```python
from build123d import *

# Parameters (mm, degrees)
SKETCH1_W             = 40
SKETCH1_H             = 30
BOSS_EXTRUDE1_DEPTH   = 400
BOSS_EXTRUDE1_2_DEPTH = 400
BOSS_EXTRUDE2_REACH   = 553.928
SKETCH2_W             = 40
SKETCH2_H             = 30
SKETCH3_W             = 40
SKETCH3_H             = 40
BOSS_EXTRUDE3_DEPTH   = 250
SKETCH4_W             = 40
SKETCH4_H             = 30
BOSS_EXTRUDE4_DEPTH   = 270
SKETCH5_W             = 40
SKETCH5_H             = 40
BOSS_EXTRUDE5_DEPTH   = 250
SKETCH6_W             = 40
SKETCH6_H             = 40
BOSS_EXTRUDE6_DEPTH   = 310


with BuildPart() as part:
    # Sketch1 → Boss-Extrude1 (new body)
    with BuildSketch(Plane.XY):
        Rectangle(SKETCH1_W, SKETCH1_H)
    extrude(amount=BOSS_EXTRUDE1_DEPTH)


with BuildPart() as body_2:
    # Sketch1 → Boss-Extrude1 2 (new body)
    with BuildSketch(Plane.XY):
        with Locations((380, 0)):
            Rectangle(SKETCH1_W, SKETCH1_H)
    extrude(amount=BOSS_EXTRUDE1_2_DEPTH)

    # Sketch2 → Boss-Extrude2 (add, up to next)
    with BuildSketch(Plane(origin=(20, 0, 0), x_dir=(0, 0, -1), z_dir=(1, 0, 0)), mode=Mode.PRIVATE) as boss_extrude2_sk1:
        with Locations((-380, 0)):
            Rectangle(SKETCH2_W, SKETCH2_H)
    boss_extrude2_tool1 = extrude(boss_extrude2_sk1.sketch, amount=BOSS_EXTRUDE2_REACH, mode=Mode.PRIVATE) - body_2.part
    # Sketch2 → Boss-Extrude2 (add, up to next)
    with BuildSketch(Plane(origin=(20, 0, 0), x_dir=(0, 0, -1), z_dir=(1, 0, 0)), mode=Mode.PRIVATE) as boss_extrude2_sk2:
        with Locations((-290, 0)):
            Rectangle(SKETCH2_W, SKETCH2_H)
    boss_extrude2_tool2 = extrude(boss_extrude2_sk2.sketch, amount=BOSS_EXTRUDE2_REACH, mode=Mode.PRIVATE) - body_2.part
    # Sketch2 → Boss-Extrude2 (add, up to next)
    with BuildSketch(Plane(origin=(20, 0, 0), x_dir=(0, 0, -1), z_dir=(1, 0, 0)), mode=Mode.PRIVATE) as boss_extrude2_sk3:
        with Locations((-110, 0)):
            Rectangle(SKETCH2_W, SKETCH2_H)
    boss_extrude2_tool3 = extrude(boss_extrude2_sk3.sketch, amount=BOSS_EXTRUDE2_REACH, mode=Mode.PRIVATE) - body_2.part
    # Sketch2 → Boss-Extrude2 (add, up to next)
    with BuildSketch(Plane(origin=(20, 0, 0), x_dir=(0, 0, -1), z_dir=(1, 0, 0)), mode=Mode.PRIVATE) as boss_extrude2_sk4:
        with Locations((-20, 0)):
            Rectangle(SKETCH2_W, SKETCH2_H)
    boss_extrude2_tool4 = extrude(boss_extrude2_sk4.sketch, amount=BOSS_EXTRUDE2_REACH, mode=Mode.PRIVATE) - body_2.part
    # Sketch2 → Boss-Extrude2 (add, up to next)
    with BuildSketch(Plane(origin=(20, 0, 0), x_dir=(0, 0, -1), z_dir=(1, 0, 0)), mode=Mode.PRIVATE) as boss_extrude2_sk5:
        with Locations((-200, 0)):
            Rectangle(SKETCH2_W, SKETCH2_H)
    boss_extrude2_tool5 = extrude(boss_extrude2_sk5.sketch, amount=BOSS_EXTRUDE2_REACH, mode=Mode.PRIVATE) - body_2.part

    add(part.part)  # Boss-Extrude2 merges part
    add(boss_extrude2_tool1.solids().sort_by_distance((20, 0, 380))[0])
    add(boss_extrude2_tool2.solids().sort_by_distance((20, 0, 290))[0])
    add(boss_extrude2_tool3.solids().sort_by_distance((20, 0, 110))[0])
    add(boss_extrude2_tool4.solids().sort_by_distance((20, 0, 20))[0])
    add(boss_extrude2_tool5.solids().sort_by_distance((20, 0, 200))[0])

    # Sketch3 → Boss-Extrude3 (add)
    with BuildSketch(Plane.XZ.offset(15)):
        with Locations((0, 380)):
            Rectangle(SKETCH3_W, SKETCH3_H)
        with Locations((0, 20)):
            Rectangle(SKETCH3_W, SKETCH3_H)
        with Locations((380, 380)):
            Rectangle(SKETCH3_W, SKETCH3_H)
        with Locations((380, 20)):
            Rectangle(SKETCH3_W, SKETCH3_H)
    extrude(amount=BOSS_EXTRUDE3_DEPTH)

    # Sketch4 → Boss-Extrude4 (add)
    with BuildSketch(Plane(origin=(0, 0, 0), x_dir=(-1, 0, 0), z_dir=(0, 0, -1))):
        with Locations((-380, 0)):
            Rectangle(SKETCH4_W, SKETCH4_H)
        Rectangle(SKETCH4_W, SKETCH4_H)
    extrude(amount=BOSS_EXTRUDE4_DEPTH)

    # Sketch5 → Boss-Extrude5 (add)
    with BuildSketch(Plane.XZ.offset(15)):
        with Locations((0, -250)):
            Rectangle(SKETCH5_W, SKETCH5_H)
        with Locations((380, -250)):
            Rectangle(SKETCH5_W, SKETCH5_H)
    extrude(amount=BOSS_EXTRUDE5_DEPTH)

    # Sketch6 → Boss-Extrude6 (add)
    with BuildSketch(Plane(origin=(0, 15, 0), x_dir=(1, 0, 0), z_dir=(0, 1, 0))):
        with Locations((0, 250)):
            Rectangle(SKETCH6_W, SKETCH6_H)
        with Locations((380, 250)):
            Rectangle(SKETCH6_W, SKETCH6_H)
        with Locations((0, 20)):
            Rectangle(SKETCH6_W, SKETCH6_H)
        with Locations((380, 20)):
            Rectangle(SKETCH6_W, SKETCH6_H)
    extrude(amount=BOSS_EXTRUDE6_DEPTH)


solid = body_2.part
```
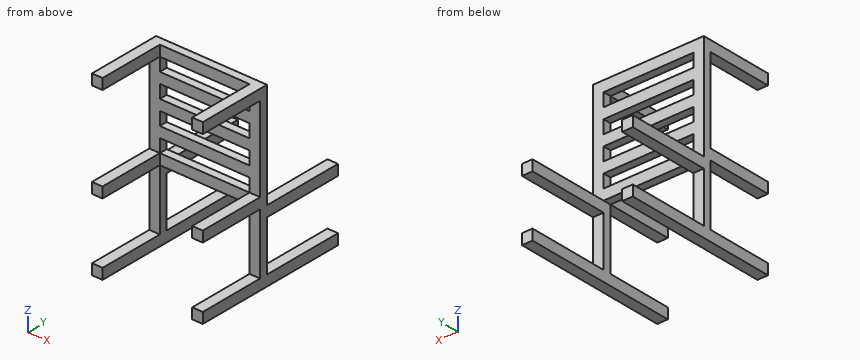
Model file for the job. Use its own axes, mm. Coordinates: 2 decimals unless noted, no trailing zeros. Write each loop counter-clockwise with the first axis right and the second up, starting at its lowest first coordinate (ties: lowest second). Pieces come first, ordered by that corner, then holes. Notation, with made-up numbers: (-9, -27.75) - (46, -27.75) arc R25 ccw to (46, 3.25) - close; hole circle Ø10 at (-9, 83). An arc over 180 degrees is marked (long way). Use a Markdown table: item, result. Add a question column.
Item 1: Drill centre lines: line 1 along Z through (x, y) = (383, -108); line 2 along X through (y, z) = (53, -243); line 3 along Z through (x, y) = (383.5, 107.5). Where is each one in solid material? Low to high.
Item 2: Band-saw the part on C-C, the plane x = 100. Write the cut outline in (y, z), and give its area (3 significant figures).
Item 3: Band-saw the part on A-A, the plane z = 152. Write the cut outline in (x, y), and give its area (3 significant figures).
Item 4: Drop flat-ended pins along their axis: pin 1 (20 mm diameter, centred on x = 370, y = 194.5, fed in from +Z); pin 2 (6 mm diameter, centred on x = 76.5, z = 273, fed in from +Y); pin 3 (9 mm diameter, centred on x = 263.5, y = 2.5, fed in from -Z). Give the stop position or say it passes through.
Item 5: Band-saw the part on D-D, the plane y = 2.5. Write the cut outline in (x, z).
Item 6: Band-saw the part on B-B, the plane y = -184. Write the cut outline in (x, z), and give its area (3 significant figures).
A:
| question | item | result |
|---|---|---|
| 1 | line 1 | z = -270 to -230, 0 to 40, 360 to 400 |
| 1 | line 2 | x = -20 to 20, 360 to 400 |
| 1 | line 3 | z = -270 to -230, -40 to 0 |
| 2 | outline | (-15, 0) - (15, 0) - (15, 40) - (-15, 40) - close; (-15, 90) - (15, 90) - (15, 130) - (-15, 130) - close; (-15, 180) - (15, 180) - (15, 220) - (-15, 220) - close; (-15, 270) - (15, 270) - (15, 310) - (-15, 310) - close; (-15, 360) - (15, 360) - (15, 400) - (-15, 400) - close |
| 2 | area | 6,000 mm² |
| 3 | outline | (-20, -15) - (20, -15) - (20, 15) - (-20, 15) - close; (360, -15) - (400, -15) - (400, 15) - (360, 15) - close |
| 3 | area | 2,400 mm² |
| 4 | pin 1 | stops at z = 0 |
| 4 | pin 2 | stops at y = 15 |
| 4 | pin 3 | stops at z = 0 |
| 5 | outline | (-20, -270) - (20, -270) - (20, 0) - (360, 0) - (360, -270) - (400, -270) - (400, 400) - (-20, 400) - close; hole (20, 40) - (360, 40) - (360, 90) - (20, 90) - close; hole (20, 130) - (360, 130) - (360, 180) - (20, 180) - close; hole (20, 220) - (360, 220) - (360, 270) - (20, 270) - close; hole (20, 310) - (360, 310) - (360, 360) - (20, 360) - close |
| 6 | outline | (-20, -270) - (20, -270) - (20, -230) - (-20, -230) - close; (-20, 0) - (20, 0) - (20, 40) - (-20, 40) - close; (-20, 360) - (20, 360) - (20, 400) - (-20, 400) - close; (360, -270) - (400, -270) - (400, -230) - (360, -230) - close; (360, 0) - (400, 0) - (400, 40) - (360, 40) - close; (360, 360) - (400, 360) - (400, 400) - (360, 400) - close |
| 6 | area | 9,600 mm² |
